Check sheet for the modelled part. Datum: model origin and axes. Units: mm. A direction names the side the tool comes from. Give positions to 0.01 mm unless a question says otherwise; leave off trailing zeros. Loops run counter-clockwise (first coordinate to the right, second up) from the corner with the lowest first, then second, coordinate; pieces in that order, holes last. Notation, with made-up numbers: M 31.5,8 L 73.5,8 A12 ccw 73.5,23 Z; hole C -31.75,86 d9. An arc over 180 degrees is marked long. Write each question's results on one line, items separated by ' | '. Start each with the question number.
1. Go/stop test with a flat-tipped pin: pin 1 (4.5 mm diameter, centred on x = 5, y = 2, fed in from -Z). Record where the tip stops, or that it passes through.
2. Sectioned sample at A-A on x = 19. Record the cut outline in (y, z), and give its area (3 significant figures).
3. Material ranges on line 1 along X through (y, z) = (-2, 13.6); line 2 along X through (y, z) = (23, 13.4); line 3 along X through (y, z) = (6.5, 14), recorded low to high.
4. Draft check along Y on faces 1 (the flat face through (-9, 27.324, 13)), 2 (the cylindrical face through (-43.843, -21.9, 13.483)), 3 (the flat face through (-48.635, 1, 13)). Enter one of: pulls with the +Y half, pulls with the -Y half, needs draft (parallel to the pull), parting line crosses it, or undercut.
5. Tool access check on faces 4 (the flat face through (5.315, -1, 14)), 5 (the flat face through (-10, 1, 14.243)). Record the directions out of +Z, -Z, +X, -X, +Y, -Y that give a thin tool (end or side, any length) a straight path to the whole face; none if there is none.
6. Sectioned sample at B-B on y = -7. Record the cut outline in (x, z).
7. Sectioned sample at C-C on z = 14. Record the cut outline in (x, y), and give its area (3 significant figures).
```python
from build123d import *

# Parameters (mm, degrees)
SKETCH1_R           = 1.25
SKETCH1_W           = 10.925559674
SKETCH1_H           = 29.413801758
BOSS_EXTRUDE1_DEPTH = 1.5
CUT_EXTRUDE1_DEPTH  = 2.5
CUT_EXTRUDE6_START  = -1.5
CUT_EXTRUDE6_DEPTH  = 1
FILLET1_R           = 1


# Read off the part's stored shape, not the designer's step: Cut-Extrude6
with BuildPart() as part:
    # Sketch1 → Boss-Extrude1 (new body)
    with BuildSketch(Plane.XY.offset(12.743078908)):
        with BuildLine():
            Line((29.564858702, -24.475637141), (29.564858702, 25.924362859))
            ThreePointArc((29.564858702, 25.924362859), (29.154808195, 26.914312353), (28.164858702, 27.324362859))
            Line((28.164858702, 27.324362859), (-47.235141298, 27.324362859))
            ThreePointArc((-47.235141298, 27.324362859), (-48.225090792, 26.914312353), (-48.635141298, 25.924362859))
            Line((-48.635141298, 25.924362859), (-48.635141298, -24.475637141))
            ThreePointArc((-48.635141298, -24.475637141), (-48.225090792, -25.465586635), (-47.235141298, -25.875637141))
            Line((-47.235141298, -25.875637141), (28.164858702, -25.875637141))
            ThreePointArc((28.164858702, -25.875637141), (29.154808195, -25.465586635), (29.564858702, -24.475637141))
        make_face()
        with Locations((-45.035141298, -22.275637141)):
            Circle(SKETCH1_R, mode=Mode.SUBTRACT)
        with Locations((-45.035141298, 23.724362859)):
            Circle(SKETCH1_R, mode=Mode.SUBTRACT)
        with Locations((25.964858702, -22.275637141)):
            Circle(SKETCH1_R, mode=Mode.SUBTRACT)
        with Locations((25.964858702, 23.724362859)):
            Circle(SKETCH1_R, mode=Mode.SUBTRACT)
        with Locations((17.892390482, 1.364242189)):
            Rectangle(SKETCH1_W, SKETCH1_H, mode=Mode.SUBTRACT)
    extrude(amount=BOSS_EXTRUDE1_DEPTH)

    # Sketch2 → Cut-Extrude1 (cut)
    with BuildSketch(Plane.XY.offset(14.243078908)):
        with BuildLine():
            ThreePointArc((8.614677666, 1.323444705), (8.416130841, 1.254039367), (8.214677666, 1.193586405))
            Line((8.214677666, 1.193586405), (8.214677666, -4.275635234))
            Line((8.214677666, -4.275635234), (8.614677666, -4.275635234))
            Line((8.614677666, -4.275635234), (8.614677666, 1.323444705))
        make_face()
        with BuildLine():
            ThreePointArc((11.464858702, 5.724364766), (10.684682981, 3.191992888), (8.614677666, 1.537707701))
            Line((8.614677666, 1.537707701), (8.614677666, 1.323444705))
            ThreePointArc((8.614677666, 1.323444705), (10.827768818, 3.047066607), (11.664858702, 5.724364766))
            ThreePointArc((11.664858702, 5.724364766), (4.287560542, 9.587274882), (5.315039737, 1.323444705))
            Line((5.315039737, 1.323444705), (5.315039737, 1.537707701))
            ThreePointArc((5.315039737, 1.537707701), (4.432486823, 9.444189046), (11.464858702, 5.724364766))
        make_face()
        with BuildLine():
            ThreePointArc((8.614677666, 1.537707701), (8.416278493, 1.464860031), (8.214677666, 1.401408306))
            Line((8.214677666, 1.401408306), (8.214677666, 1.193586405))
            ThreePointArc((8.214677666, 1.193586405), (8.416130841, 1.254039367), (8.614677666, 1.323444705))
            Line((8.614677666, 1.323444705), (8.614677666, 1.537707701))
        make_face()
        with BuildLine():
            Line((5.715039737, -4.275635234), (5.715039737, 1.193586405))
            ThreePointArc((5.715039737, 1.193586405), (5.513586562, 1.254039367), (5.315039737, 1.323444705))
            Line((5.315039737, 1.323444705), (5.315039737, -4.275635234))
            Line((5.315039737, -4.275635234), (5.715039737, -4.275635234))
        make_face()
        with BuildLine():
            Line((5.715039737, 1.193586405), (5.715039737, 1.401408306))
            ThreePointArc((5.715039737, 1.401408306), (5.51343891, 1.464860031), (5.315039737, 1.537707701))
            Line((5.315039737, 1.537707701), (5.315039737, 1.323444705))
            ThreePointArc((5.315039737, 1.323444705), (5.513586562, 1.254039367), (5.715039737, 1.193586405))
        make_face()
    extrude(amount=-CUT_EXTRUDE1_DEPTH, mode=Mode.SUBTRACT)

    # Cut-Extrude6 outline → Cut-Extrude6 (cut)
    with BuildSketch(Plane.XY.offset(14.243078908).offset(CUT_EXTRUDE6_START)):
        with BuildLine():
            Line((5.715039737, 1.401408306), (5.715039737, -4.275635234))
            Line((5.715039737, -4.275635234), (8.214677666, -4.275635234))
            Line((8.214677666, -4.275635234), (8.214677666, 1.401408306))
            ThreePointArc((8.214677666, 1.401408306), (6.964858701, 10.224364766), (5.715039737, 1.401408306))
        make_face()
    extrude(amount=CUT_EXTRUDE6_DEPTH, mode=Mode.SUBTRACT)

    # Fillet1
    fillet1_edges = [part.edges().sort_by_distance(p)[0] for p in [
        (6.964858701, -4.275635234, 13.743078908),
    ]]
    fillet(fillet1_edges, radius=FILLET1_R - 0.0001)  # a hair under: the kernel refuses the full size


solid = part.part
```
Output values:
1) pin 1: z = 12.74
2) outline: M -25.88,12.74 L -13.34,12.74 L -13.34,14.24 L -25.88,14.24 Z; M 16.07,12.74 L 27.32,12.74 L 27.32,14.24 L 16.07,14.24 Z | area: 35.7 mm2
3) line 1: -48.64 to 5.32, 8.61 to 12.43, 23.36 to 29.56 | line 2: -48.64 to -46.05, -44.02 to 24.95, 26.98 to 29.56 | line 3: -48.64 to 2.33, 2.53 to 11.4, 11.6 to 12.43, 23.36 to 29.56
4) face 1: pulls with the +Y half | face 2: undercut | face 3: needs draft
5) face 4: +Z, -Z | face 5: +Z, +X, -X, +Y, -Y
6) outline: M -48.64,12.74 L 12.43,12.74 L 12.43,14.24 L -48.64,14.24 Z; M 23.36,12.74 L 29.56,12.74 L 29.56,14.24 L 23.36,14.24 Z
7) outline: M -48.64,-24.48 A1.4 ccw -47.24,-25.88 L 28.16,-25.88 A1.4 ccw 29.56,-24.48 L 29.56,25.92 A1.4 ccw 28.16,27.32 L -47.24,27.32 A1.4 ccw -48.64,25.92 Z; hole C -45.04,-22.28 d2.5; hole C -45.04,23.72 d2.5; hole M 5.32,-4.28 L 5.72,-4.28 L 5.72,1.4 A4.5 cw long 8.21,1.4 L 8.21,-4.28 L 8.61,-4.28 L 8.61,1.32 A4.7 ccw long 5.32,1.32 Z; hole M 12.43,-13.34 L 23.36,-13.34 L 23.36,16.07 L 12.43,16.07 Z; hole C 25.96,-22.28 d2.5; hole C 25.96,23.72 d2.5 | area: 3,810 mm2
